Check sheet for the modelled part. Datum: model origin and axes. Units: mm. Face numbers are marked on the shaded views. A direction names the side the tool comes from. Round coordinates to 2 decimals unless told otherwise and drop trailing zeros. Write each loop counter-clockwise with the first axis right and the second up, starting at its lowest first coordinate (ties: lowest second). Pieces come first, ordered by that corner, then holes.
Item 1: Tool access check on the marked faces 1 and 2. Record the directions out of +Z, -Z, +X, -X, +Y, -Y that give a thin tool (end or side, any length) a straight path to the whole face; none if there is none.
Item 2: Cross-section at C-C on x = 20. Enter the section's corners in (y, z), plus the area to 3 significant figures.
Item 3: Cross-section at B-B on z = 6.5. Enter the section's corners in (x, y), plus the area to 3 significant figures.
Item 4: Material ranges on line 1 (Y direction, x = 10, z = 37.5); line 2 (X direction, y = -2, z = 52); line 3 (Y direction, x = 30, z = 66.5), recorded low to high.
Item 5: Cross-section at D-D on y = -16.5. Enter the section's corners in (x, z).
Item 6: Cross-section at A-A on x = 32. Enter the section's corners in (y, z).
Item 7: Go/stop test with flat-tipped pins: pin 1 Ø12 at (y, z) = (12.5, 65.5) entering from -X; pin 2 Ø11 at (y, z) = (-6, 24.5) entering from +X. Record where each tip stops, or that it passes through.
Autodesk Inventor part; units mm, degrees
ref_plane "Начальная плоскость" through (0, 0, 0) normal (0, 0, 1) x (1, 0, 0)
ref_plane "Конечная плоскость" through (0, 0, 86.12) normal (0, 0, 1) x (1, 0, 0)
ref_plane "РабПлоскость8" through (18, 177.5, 86.12) normal (0, 0, 1) x (1, 0, 0)
ref_plane "Начальная плоскость" through (0, 0, 0) normal (0, 0, 1) x (1, 0, 0)
ref_plane "Конечная плоскость" through (0, 0, 86.12) normal (0, 0, 1) x (1, 0, 0)
sketch "Эскиз" plane through (0, 0, 0) normal (0, 0, 1) x (1, 0, 0)
  line L0 (36, -32.5) -> (0, -32.5)
  line L1 (36, -32.5) -> (36, -28.696)
  line L2 (33.6994, -26.2039) -> (9.9215, -24.3017)
  line L3 (4.4, -18.3208) -> (4.4, 18.3208)
  line L4 (33.6994, 26.2039) -> (9.9215, 24.3017)
  line L5 (36, 28.696) -> (36, 32.5)
  line L6 (0, 32.5) -> (36, 32.5)
  line L7 (0, -32.5) -> (0, 32.5)
  arc A0 (4.4, -18.3208) -> (9.9215, -24.3017) centre (10.4, -18.3208) ccw
  arc A1 (9.9215, 24.3017) -> (4.4, 18.3208) centre (10.4, 18.3208) ccw
  arc A2 (36, -28.696) -> (33.6994, -26.2039) centre (33.5, -28.696) ccw
  arc A3 (33.6994, 26.2039) -> (36, 28.696) centre (33.5, 28.696) ccw
  line L8 (0, 45.5) -> (0, -45.5) construction
  line L9 (-7.2974, 0) -> (43.7847, 0) construction
  point P0 (36, -26.388)
  point P1 (4.4, -23.86)
  point P2 (4.4, 23.86)
  point P3 (36, 26.388)
  dimension "d3" = 36
  dimension "d5" = 4.4
  dimension "d7" = 65
  dimension "d9" = 8.64
  dimension "d11" = 8.64
  dimension "d13" = 6.112
  dimension "d15" = 6.112
  dimension "d22" = 6
  dimension "d23" = 2.5
  dimension "d24" = 32.5
  dimension "d25" = 0
extrude "Тело" add sketch "Эскиз" along normal up to surface (86.12 mm away) from surface at 0
sketch "Sketch3" plane through (0, 0, 0) normal (0, 0, 1) x (1, 0, 0)
  line L0 (0, 0) -> (10, 0)
ref_plane "Work Plane7" through (0, 0, 0) normal (0, -1, 0) x (1, 0, 0)
sketch "Sketch4" plane through (0, 0, 0) normal (0, -1, 0) x (1, 0, 0)
  line L0 (-2, 0) -> (12, 0)
  line L1 (-2, 86.12) -> (12, 86.12)
  dimension "d29" = 86.12
ref_plane "РабПлоскость8" through (18, 177.5, 86.12) normal (0, 0, 1) x (1, 0, 0)
split "Разделение1" plane through (18, 177.5, 86.12) removes the side toward (0, 0, 1)
ref_plane "РабПлоскость9" through (546.459, 0, 0) normal (0, 0, -1) x (-1, 0, 0)
split "Разделение2" plane through (546.459, 0, 0) removes the side toward (0, 0, -1)
equation "\"d3\" = b"
equation "\"d7\" = ParH"
equation "\"d22\" = R"
equation "\"d23\" = R1"
equation "\"d24\" = 0.5 * d7"
equation "\"d16\" = G_L"
equation "\"R1\" = 2.5"
equation "\"R\" = 6"
equation "\"t1\" = 4.4"
equation "\"t2\" = 7.2"
equation "\"ParH\" = 65"
equation "\"b\" = 36"
equation "\"msp_x1\" = 0.04 * b"
equation "\"msp_x2\" = -0.08 * t1 + 0.04 * b"
equation "\"G_L\" = d29"
equation "\"ex\" = 0"
equation "\"G_OFFSET_START\" = 0"
equation "\"G_OFFSET_END\" = 0"
equation "\"d27\" = G_OFFSET_END + B_L"
equation "\"B_L\" = 86.12"
properties part number "Швеллер 6.5U-86,12 ГОСТ 8240-97" material "Сталь, мягкая, сварочная"
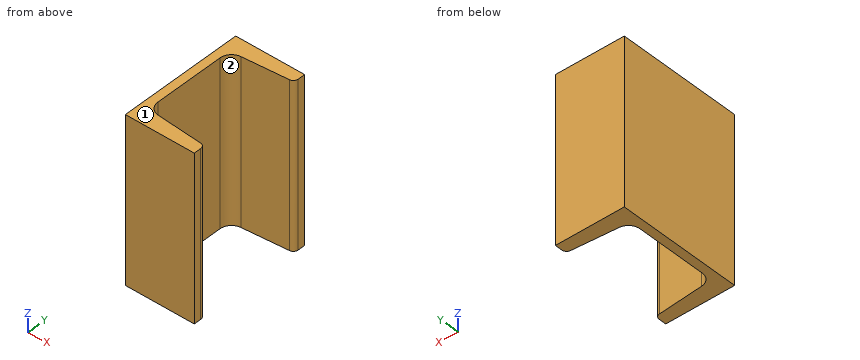
Response values:
1. face 1: +Z, +X, -X, +Y, -Y
1. face 2: +Z, -Z, +X
2. outline: (-32.5, 0) - (-25.11, 0) - (-25.11, 86.12) - (-32.5, 86.12) - close; (25.11, 0) - (32.5, 0) - (32.5, 86.12) - (25.11, 86.12) - close
2. area: 1,270 mm2
3. outline: (0, -32.5) - (36, -32.5) - (36, -28.7) arc R2.5 ccw to (33.7, -26.2) - (9.92, -24.3) arc R6 cw to (4.4, -18.32) - (4.4, 18.32) arc R6 cw to (9.92, 24.3) - (33.7, 26.2) arc R2.5 ccw to (36, 28.7) - (36, 32.5) - (0, 32.5) - close
3. area: 763 mm2
4. line 1: y = -32.5 to -24.31, 24.31 to 32.5
4. line 2: x = 0 to 4.4
4. line 3: y = -32.5 to -25.91, 25.91 to 32.5
5. outline: (0, 0) - (4.4, 0) - (4.4, 86.12) - (0, 86.12) - close
6. outline: (-32.5, 0) - (-26.07, 0) - (-26.07, 86.12) - (-32.5, 86.12) - close; (26.07, 0) - (32.5, 0) - (32.5, 86.12) - (26.07, 86.12) - close
7. pin 1: stops at x = 0
7. pin 2: stops at x = 4.4
